Could you check a few things on this drawing? It's one solid part, dimensions in mm from its lowest x, y, z. A direction names the side the tool comes from. Round coordinates to 2 decimals unless told otherwise and drop trailing zeros. Order: outer loops, then holes, each group sorted by start corner. A loop starts at its lowest first (then second) coordinate and runs counter-clockwise, first axis right, second up. Notation, with made-up numbers: (0, -39) -> (43, -39) arc R21 ccw to (43, -16) -> close; hole circle Ø4 at (-29.75, 21.25). An arc over 180 degrees is marked (long way). Use a Markdown table: item, result. Add a question column.
(1) I'm going to push flat-ended pins straight in: P1, Ø2.5, axis at x = 20, z = 12, coming from the -Y side; P2, Ø4, axis at x = 6, z = 17.5, coming from the +Y side; P3, Ø6, axis at x = 17, y = 10, coming from the +Z side. Where does each tip first touch, or does it pass through?
(2) If I drill on probe 1 along Y at (x, z) = (38.2, 3.5); probe 2 along Y at (x, z) = (37.6, 22.5); probe 3 along X at (y, z) = (1, 12.5), over which ranges is the centre line in solid material (lowest first)?
(3) I want a section at C-C, the plane z = 16.25. Please give me the cut outline in (x, y), then the cut area to 3 significant figures.
(4) On a 3-axis mill with a long thin cutter (end or side, diameter ignored), from which of +Z, -Z, +X, -X, +Y, -Y can I reach the whole of each face in a straight line? I mean the marked faces 1, 2, 3, 4 and 5. Say none if no direction works.
(5) I want a section at A-A, the plane z = 22.5. Please give me the cut outline in (x, y).
(6) I want a section at D-D, the plane y = 28. Please give me the cut outline in (x, z).
(7) I want a section at B-B, the plane y = 15.5. Please give me the cut outline in (x, z).
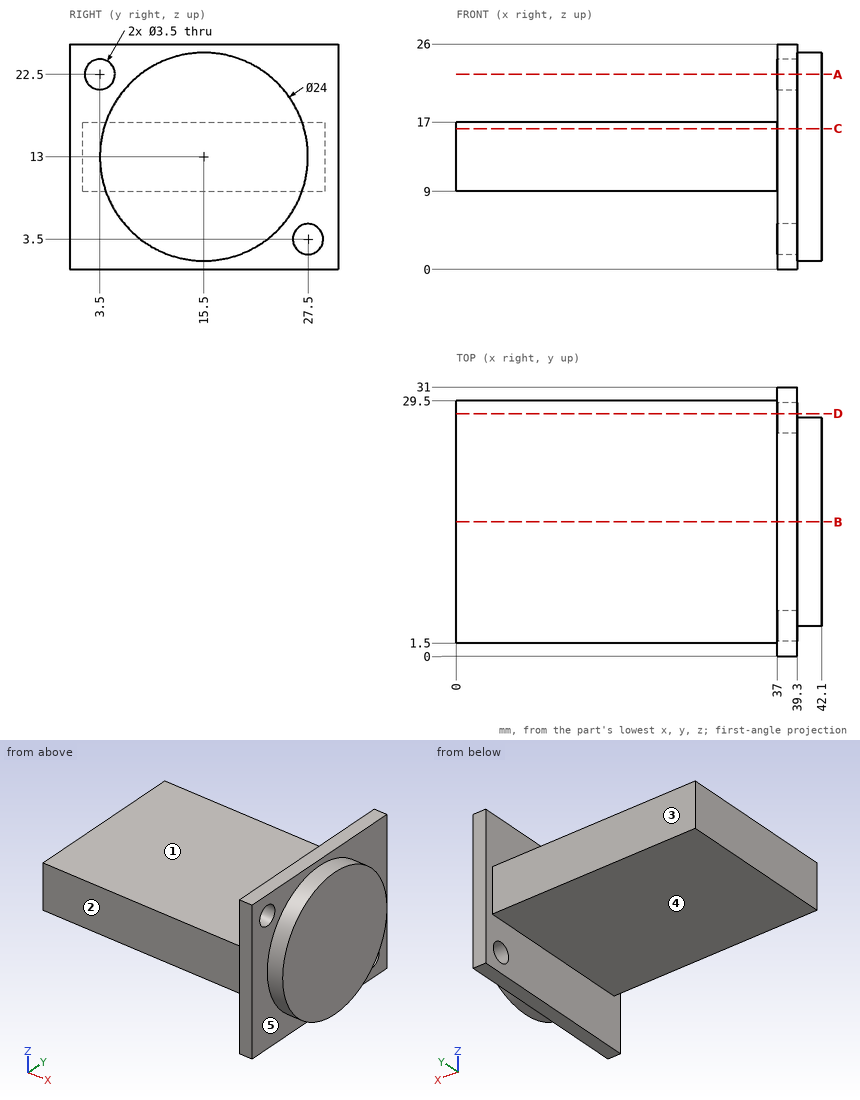
Taken from the geometry:
| question | item | result |
|---|---|---|
| 1 | P1 | stops at y = 1.5 |
| 1 | P2 | stops at y = 29.5 |
| 1 | P3 | stops at z = 17 |
| 2 | probe 1 | y = 0 to 25.75, 29.25 to 31 |
| 2 | probe 2 | y = 0 to 1.75, 5.25 to 31 |
| 2 | probe 3 | x = 37 to 39.3 |
| 3 | outline | (0, 1.5) -> (37, 1.5) -> (37, 0) -> (39.3, 0) -> (39.3, 3.95) -> (42.1, 3.95) -> (42.1, 27.05) -> (39.3, 27.05) -> (39.3, 31) -> (37, 31) -> (37, 29.5) -> (0, 29.5) -> close |
| 3 | area | 1,170 mm2 |
| 4 | face 1 | +Z, -X, +Y, -Y |
| 4 | face 2 | +Z, -Z, -X, -Y |
| 4 | face 3 | +Z, -Z, -X, +Y |
| 4 | face 4 | -Z, -X, +Y, -Y |
| 4 | face 5 | +X |
| 5 | outline | (37, 0) -> (39.3, 0) -> (39.3, 1.75) -> (37, 1.75) -> close; (37, 5.25) -> (39.3, 5.25) -> (39.3, 8.17) -> (42.1, 8.17) -> (42.1, 22.83) -> (39.3, 22.83) -> (39.3, 31) -> (37, 31) -> close |
| 6 | outline | (0, 9) -> (37, 9) -> (37, 5.18) -> (39.3, 5.18) -> (39.3, 26) -> (37, 26) -> (37, 17) -> (0, 17) -> close; (37, 0) -> (39.3, 0) -> (39.3, 1.82) -> (37, 1.82) -> close |
| 7 | outline | (0, 9) -> (37, 9) -> (37, 0) -> (39.3, 0) -> (39.3, 1) -> (42.1, 1) -> (42.1, 25) -> (39.3, 25) -> (39.3, 26) -> (37, 26) -> (37, 17) -> (0, 17) -> close |
